```python
from build123d import *

# Parameters (mm, degrees)
CYLINDER_R         = 10
CYLINDER_DEPTH     = 14
POCKET_DEPTH       = 10
SKETCH001_R        = 2
POCKET001_DEPTH    = 14
POLARPATTERN_COUNT = 8


with BuildPart() as part:
    # Cylinder → Cylinder (new body)
    with BuildSketch(Plane.XY):
        Circle(CYLINDER_R)
    extrude(amount=CYLINDER_DEPTH)

    # Sketch → Pocket (cut)
    with BuildSketch(Plane(origin=(0, 0, 0), x_dir=(1, 0, 0), z_dir=(0, 0, -1))):
        with BuildLine():
            ThreePointArc((-1.5, -2.826659), (3.2, 0), (-1.5, 2.826659))
            Line((-1.5, -2.826659), (-1.5, 2.826659))
        make_face()
    extrude(amount=-POCKET_DEPTH, mode=Mode.SUBTRACT)

    # Sketch001 → Pocket001 (cut)
    with BuildSketch(Plane(origin=(0, 0, 0), x_dir=(1, 0, 0), z_dir=(0, 0, -1))):
        with Locations((-11, 0)):
            Circle(SKETCH001_R)
    pocket001 = extrude(amount=-POCKET001_DEPTH, mode=Mode.SUBTRACT)

    # PolarPattern: Pocket001 ×8 about axis
    polarpattern_axis = Axis((0, 0, 0), (0, 0, -1))
    for i in range(1, POLARPATTERN_COUNT):
        add(pocket001.rotate(polarpattern_axis, i * 360 / POLARPATTERN_COUNT), mode=Mode.SUBTRACT)


solid = part.part
```
Geometry: final body of the model. Coordinates: model frame, mm. A direction names the side the tool comes from. Give positions to 0.01 mm unless a question says otherwise; leave off trailing zeros. Write each loop counter-clockwise with the first axis right and the second up, starting at its lowest first coordinate (ties: lowest second). Pieces come first, ordered by that corner, then holes.
1. Reachability of faces 1 (the flat face through (-1.5, 0, 5)), 2 (the cylindrical face through (-9.227, 3.856, 6.902)) from +Z, -Z, +X, -X, +Y, -Y: full face, straight path, thin tool, end or side. Return the list, or none.
2. Section query C-C, the plane y = 0. Return loops of the section in (x, z).
3. Section query A-A, the plane z = 3.25. Return loops of the section in (x, y), then the cut area to 3 significant figures.
4. Section query D-D, the plane x = 3.75. Return loops of the section in (y, z), then the cut area to 3 significant figures.
5. Draft query along Y for faces 3 (the cylindrical face through (9.25, 3.8, 6.9)), 4 (the cylindrical face through (-3.856, -9.227, 6.902)), 5 (the cylindrical face through (6.345, -6.383, 6.902)). Return one class per face: released by +Y, released by -Y, zero draft, split by the parting line, or undercut.
6. Line query: probe 1 along Y at (x, z) = (0, 2.5); probe 2 along Z at (x, y) = (1.5, -0.5); probe 3 along X at (y, z) = (0.25, 8.5). Output: solid intervals per line, ascending.
7. Section query B-B, the plane x = 0. Return loops of the section in (y, z), then the cut area to 3 significant figures.
8. Pin query (flat end, axial travel): P1, Ø4, axis at x = -2.5, y = -0.5, coming from the -Z side; P2, Ø1.5, axis at y = 5, z = 5.5, coming from the -X side; P3, Ø3, axis at x = 6, z = 2.5, coming from the +Y side; P4, Ø1.5, axis at y = -6.5, z = 9.5, coming from the +X side. Return the tip coordinate at first contact, or that it passes through.
Computed:
1. face 1: -Z
1. face 2: +Z, -Z, -X, +Y
2. outline: (-9, 0) - (-1.5, 0) - (-1.5, 10) - (3.2, 10) - (3.2, 0) - (9, 0) - (9, 14) - (-9, 14) - close
3. outline: (-9.86, -1.65) arc R10 ccw to (-8.14, -5.81) arc R2 cw to (-5.81, -8.14) arc R10 ccw to (-1.65, -9.86) arc R2 cw to (1.65, -9.86) arc R10 ccw to (5.81, -8.14) arc R2 cw to (8.14, -5.81) arc R10 ccw to (9.86, -1.65) arc R2 cw to (9.86, 1.65) arc R10 ccw to (8.14, 5.81) arc R2 cw to (5.81, 8.14) arc R10 ccw to (1.65, 9.86) arc R2 cw to (-1.65, 9.86) arc R10 ccw to (-5.81, 8.14) arc R2 cw to (-8.14, 5.81) arc R10 ccw to (-9.86, 1.65) arc R2 cw to start; hole (-1.5, -2.83) arc R3.2 ccw (long way) to (-1.5, 2.83) - close
3. area: 270 mm2
4. outline: (-9.27, 0) - (9.27, 0) - (9.27, 14) - (-9.27, 14) - close
4. area: 260 mm2
5. face 3: released by +Y
5. face 4: released by -Y
5. face 5: undercut
6. probe 1: y = -9 to -3.2, 3.2 to 9
6. probe 2: z = 10 to 14
6. probe 3: x = -9.02 to -1.5, 3.19 to 9.02
7. outline: (-9, 0) - (-3.2, 0) - (-3.2, 10) - (3.2, 10) - (3.2, 0) - (9, 0) - (9, 14) - (-9, 14) - close
7. area: 188 mm2
8. P1: stops at z = 0
8. P2: stops at x = -9.05
8. P3: stops at y = 8.93
8. P4: stops at x = 8.18
